Solid Edge part; units mm, degrees
sketch "Sketch1" plane through (0, 0, 0) normal (0, 0, 1) x (1, 0, 0)
  line L0 (15, -71) -> (0, -71)
  line L1 (0, -71) -> (0, 0)
  line L2 (0, 0) -> (15, 0)
  line L3 (15, 0) -> (15, -71)
extrude "Protrusion1" add sketch "Sketch1" along normal blind 2
hole "Bohrung_1" at (3, -68, 2) direction (0, 0, -1) diameter 2.459 end through all
hole "Hole1" at (11.388, -63.54, 2) direction (0, 0, -1) diameter 2.459 end through all
hole "Bohrung_3" at (7.5, -7.5, 2) direction (0, 0, -1) diameter 4.3 end through all countersink diameter 9.18 countersink angle 90
hole "Hole2" at (7.5, -35.5, 2) direction (0, 0, -1) diameter 4.3 end through all countersink diameter 9.18 countersink angle 90
fillet "Verrundung_1" radius 2 4 edges at (15, 0, 1) (0, 0, 1) (15, -71, 1) (0, -71, 1)
Model file for the job. Use its own axes, mm. Round coordinates to 2 decimals unless told otherwise and drop trailing zeros. Write each loop counter-clockwise with the first axis right and the second up, starting at its lowest first coordinate (ties: lowest second). Pieces come first, ordered by that corner, then holes. Notation, with made-up numbers: M 78,32 L 104,32 A22 cw 104,51 Z; hole C 62,-4 d7. An arc over 180 degrees is marked long. Put each result on its own line as item: value.
Item 1: Cut at C-C (z = 1.55). List the corners of the cut face in (x, y), and give its area (3 significant figures).
Responses:
outline: M 0,-69 A2 ccw 2,-71 L 13,-71 A2 ccw 15,-69 L 15,-2 A2 ccw 13,0 L 2,0 A2 ccw 0,-2 Z; hole C 3,-68 d2.46; hole C 7.5,-35.5 d8.28; hole C 7.5,-7.5 d8.28; hole C 11.39,-63.54 d2.46
area: 944 mm²
Item 2: Cut at A-A (x = 7.5). List the corners of the cut face in (y, z).
Responses:
outline: M -71,0 L -38.09,0 L -40.09,2 L -71,2 Z; M -32.91,0 L -10.09,0 L -12.09,2 L -30.91,2 Z; M -4.91,0 L 0,0 L 0,2 L -2.91,2 Z
Item 3: Probe L1, parallel to Y at x = 3, z = 0.45; L2, parallel to Y at x = 7.5, z = 1.1; L3, parallel to X at y = -63.54, z = 1.45. List the from-to ranges inside material, lowest first. Write a range as from..to.
Responses:
L1: -71..-69.23, -66.77..0
L2: -71..-39.19, -31.81..-11.19, -3.81..0
L3: 0..10.16, 12.62..15
Item 4: Cut at D-D (y = -35.5). List the corners of the cut face in (x, z), and give its area (3 significant figures).
Responses:
outline: M 0,0 L 4.91,0 L 2.91,2 L 0,2 Z; M 10.09,0 L 15,0 L 15,2 L 12.09,2 Z
area: 15.6 mm²
Item 5: Mould opens along Y. For faces 1 (the flat face through (15, -35, 1)), 2 (the cylindrical face through (0.6, -0.57, 1.01)), 3 (the cylindrical face through (11.8, -64.7, 1)), 4 (the cylindrical face through (3.05, -66.77, 1.01)) say: +Y half, -Y half, draft (parallel to the pull), parting line (faces both ways), or undercut.
Responses:
face 1: draft
face 2: +Y half
face 3: undercut
face 4: undercut
Item 6: Cut at B-B (y = -68). List the corners of the cut face in (x, z).
Responses:
outline: M 0,0 L 1.77,0 L 1.77,2 L 0,2 Z; M 4.23,0 L 15,0 L 15,2 L 4.23,2 Z
